Print and shaded views of the part. All mm, measured from the part's lowest x, y and z. Coordinates: 2 decimals unless noted, no trailing zeros. Loops run counter-clockwise (first coordinate to the right, second up) from the corner with the lowest first, then second, coordinate; pieces in that order, holes last. Notation, with made-up numbers: (-25, 10) -> (5, 10) arc R22 ccw to (5, 47) -> close; hole circle Ø4 at (41, -19.5). An arc over 180 degrees is marked (long way). One line per question, with ' | ' between items. Start each with the question number.
1) Drop flat-ended pins along their axis: pin 1 (25 mm diameter, centred on y = 277, z = 27, fed in from +X); pin 2 (25 mm diameter, centred on x = 43, y = 267, fed in from +Z). Give the stop position or say it passes through.
2) Cut at A-A (x = 73.5). List the corners of the cut face in (y, z).
3) Cut at B-B (z = 37.5). List the corners of the cut face in (x, y).
4) Probe L1, parallel to Y at x = 65, z = 72; L2, parallel to Z at x = 17, y = 532.5. List the from-to ranges inside material, lowest first. Write a range as from..to.
5) Cut at C-C (x = 47). List the corners of the cut face in (y, z), plus the area to 3 significant figures.
6) Two-plate mould, pull along Y, no slides. Class the marked faces 1, 2 and 3: released by +Y, released by -Y, zero draft, split by the parting line, or undercut.
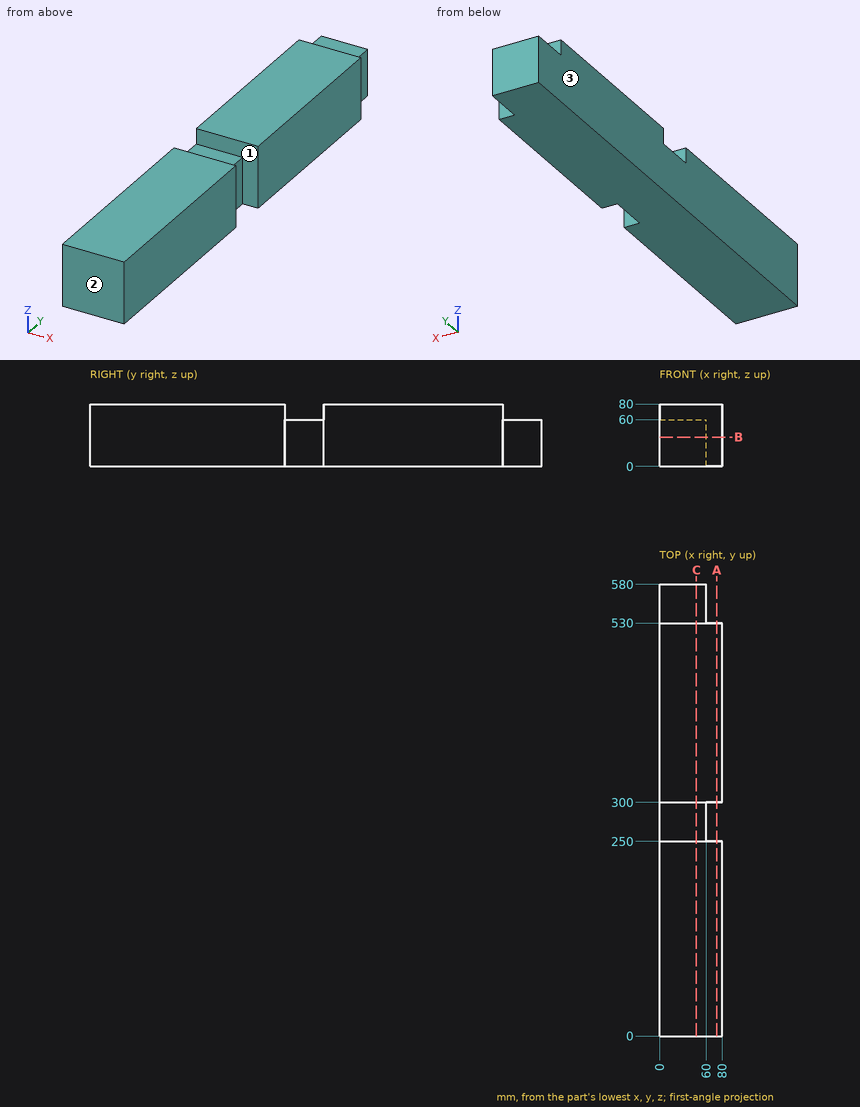
Reported:
1) pin 1: stops at x = 60 | pin 2: stops at z = 60
2) outline: (0, 0) -> (250, 0) -> (250, 80) -> (0, 80) -> close; (300, 0) -> (530, 0) -> (530, 80) -> (300, 80) -> close
3) outline: (0, 0) -> (80, 0) -> (80, 250) -> (60, 250) -> (60, 300) -> (80, 300) -> (80, 530) -> (60, 530) -> (60, 580) -> (0, 580) -> close
4) L1: y = 0..250, 300..530 | L2: z = 0..60
5) outline: (0, 0) -> (580, 0) -> (580, 60) -> (530, 60) -> (530, 80) -> (300, 80) -> (300, 60) -> (250, 60) -> (250, 80) -> (0, 80) -> close | area: 44,400 mm²
6) face 1: undercut | face 2: released by -Y | face 3: zero draft
